from build123d import *

# Parameters (mm, degrees)
SKETCH_W        = 40
SKETCH_H        = 42
SKETCH_R        = 1.6
PAD_DEPTH       = 12
SKETCH001_R     = 4.075
POCKET_DEPTH    = 42.001
SKETCH003_R     = 1.6
PAD001_DEPTH    = 40
SKETCH004_W     = 8.15
SKETCH004_H     = 42
SKETCH004_R     = 3
SKETCH004_W_2   = 7.5
POCKET001_DEPTH = 10.001
POCKET002_DEPTH = 3
POCKET003_DEPTH = 3
FILLET_R        = 4
FILLET001_R     = 3
SKETCH008_R     = 1.6
POCKET004_DEPTH = 40.001
POCKET005_DEPTH = 3
POCKET006_DEPTH = 3
POCKET007_DEPTH = 40.001


with BuildPart() as part:
    # Sketch → Pad (new body)
    with BuildSketch(Plane.XY):
        Rectangle(SKETCH_W, SKETCH_H)
        with Locations((-14.85, 11.875)):
            Circle(SKETCH_R, mode=Mode.SUBTRACT)
        with Locations((14.85, 11.875)):
            Circle(SKETCH_R, mode=Mode.SUBTRACT)
        with Locations((-14.85, -11.875)):
            Circle(SKETCH_R, mode=Mode.SUBTRACT)
        with Locations((14.85, -11.875)):
            Circle(SKETCH_R, mode=Mode.SUBTRACT)
    extrude(amount=PAD_DEPTH)

    # Sketch001 (on Face3 of Pad) → Pocket (cut, through all)
    with BuildSketch(Plane.XZ.offset(21)):
        with Locations((0, 6)):
            Circle(SKETCH001_R)
    extrude(amount=-POCKET_DEPTH, mode=Mode.SUBTRACT)

    # Sketch003 (on Face2 of Pocket) → Pad001 (join)
    with BuildSketch(Plane(origin=(-20, 0, 0), x_dir=(0, -1, 0), z_dir=(-1, 0, 0))):
        with BuildLine():
            ThreePointArc((16.875, 17), (11.875, 22), (6.875, 17))
            Line((6.875, 17), (6.875, 12))
            Line((16.875, 12), (6.875, 12))
            Line((16.875, 12), (16.875, 17))
        make_face()
        with Locations((11.875, 17)):
            Circle(SKETCH003_R, mode=Mode.SUBTRACT)
    extrude(amount=-PAD001_DEPTH)

    # Sketch004 (on Face4 of Pad001) → Pocket001 (cut, through all)
    with BuildSketch(Plane.XY.offset(12)):
        with Locations((-15.925, 0)):
            Rectangle(SKETCH004_W, SKETCH004_H)
        with Locations((-14.85, 11.875)):
            Circle(SKETCH004_R, mode=Mode.SUBTRACT)
        with Locations((15.925, 0)):
            Rectangle(SKETCH004_W, SKETCH004_H)
        Rectangle(SKETCH004_W_2, SKETCH004_H)
    extrude(amount=POCKET001_DEPTH, mode=Mode.SUBTRACT)

    # Sketch005 (on Face31 of Pocket001) → Pocket002 (cut)
    with BuildSketch(Plane.YZ.offset(11.85)):
        Polygon((-10.258419, 19.8), (-13.491581, 19.8), (-15.108162, 17), (-13.491581, 14.2), (-10.258419, 14.2), (-8.641838, 17), align=None)
    extrude(amount=-POCKET002_DEPTH, mode=Mode.SUBTRACT)

    # Sketch006 (on Face27 of Pocket002) → Pocket003 (cut)
    with BuildSketch(Plane(origin=(-11.85, 0, 0), x_dir=(0, -1, 0), z_dir=(-1, 0, 0))):
        Polygon((13.491581, 19.8), (10.258419, 19.8), (8.641838, 17), (10.258419, 14.2), (13.491581, 14.2), (15.108162, 17), align=None)
    extrude(amount=-POCKET003_DEPTH, mode=Mode.SUBTRACT)

    # Fillet
    fillet_edges = [part.edges().sort_by_distance(p)[0] for p in [
        (7.8, -16.875, 12),
        (-7.8, -16.875, 12),
        (7.8, -6.875, 12),
        (-7.8, -6.875, 12),
    ]]
    fillet(fillet_edges, radius=FILLET_R)

    # Fillet001
    fillet001_edges = [part.edges().sort_by_distance(p)[0] for p in [
        (20, -21, 6),
        (-20, -21, 6),
        (20, 21, 6),
        (-20, 21, 6),
    ]]
    fillet(fillet001_edges, radius=FILLET001_R)

    # Sketch008 (on Face5 of Fillet001) → Pocket004 (cut, through all)
    with BuildSketch(Plane(origin=(-20, 0, 0), x_dir=(0, -1, 0), z_dir=(-1, 0, 0))):
        with Locations((-4, 6)):
            Circle(SKETCH008_R)
        with Locations((4, 6)):
            Circle(SKETCH008_R)
    extrude(amount=-POCKET004_DEPTH, mode=Mode.SUBTRACT)

    # Sketch009 (on Face5 of Pocket004) → Pocket005 (cut)
    with BuildSketch(Plane(origin=(-20, 0, 0), x_dir=(0, -1, 0), z_dir=(-1, 0, 0))):
        Polygon((-2.383419, 8.8), (-5.616581, 8.8), (-7.233162, 6), (-5.616581, 3.2), (-2.383419, 3.2), (-0.766838, 6), align=None)
        Polygon((5.616581, 8.8), (2.383419, 8.8), (0.766838, 6), (2.383419, 3.2), (5.616581, 3.2), (7.233162, 6), align=None)
    extrude(amount=-POCKET005_DEPTH, mode=Mode.SUBTRACT)

    # Sketch010 (on Face42 of Pocket005) → Pocket006 (cut)
    with BuildSketch(Plane.YZ.offset(20)):
        Polygon((-2.383419, 8.8), (-5.616581, 8.8), (-7.233162, 6), (-5.616581, 3.2), (-2.383419, 3.2), (-0.766838, 6), align=None)
        Polygon((5.616581, 8.8), (2.383419, 8.8), (0.766838, 6), (2.383419, 3.2), (5.616581, 3.2), (7.233162, 6), align=None)
    extrude(amount=-POCKET006_DEPTH, mode=Mode.SUBTRACT)

    # Sketch008 (on Face5 of Fillet001) → Pocket007 (cut, through all)
    with BuildSketch(Plane(origin=(-20, 0, 0), x_dir=(0, -1, 0), z_dir=(-1, 0, 0))):
        with Locations((-4, 6)):
            Circle(SKETCH008_R)
        with Locations((4, 6)):
            Circle(SKETCH008_R)
    extrude(amount=-POCKET007_DEPTH, mode=Mode.SUBTRACT)


solid = part.part
The listing builds one solid part. Answer for the finished solid, in the listing's coordinates (mm). A direction names the side the tool comes from. Give positions to 0.01 mm unless a question says otherwise; leave off trailing zeros. Loops run counter-clockwise (first coordinate to the right, second up) from the corner with the lowest first, then second, coordinate; pieces in that order, holes last. Notation, with made-up numbers: (9.5, 48) - (27.5, 48) arc R11 ccw to (27.5, 63) - close; hole circle Ø11 at (-34, 10). An arc over 180 degrees is marked (long way). Write each question's results on one line, items separated by ' | '.
1. For a pull along Y with two mould halves and no side action, classify faces 1 (the face through (-20, 0, 6)), 2 (the face through (-4, 21, 4.6)), 3 (the face through (16.376, 12.356, 5.916)) as +Y half, -Y half, draft (parallel to the pull), parting line (faces both ways), or undercut.
Resolved:
face 1: draft | face 2: +Y half | face 3: undercut
2. Which of the six approach directions +Z, -Z, +X, -X, +Y, -Y give full straight-line access (tool end or side, diameter ignored) to faces 4 (the face through (10.4, -14.3, 15.6)), 5 (the face through (-18.521, 6.436, 4.62)), 6 (the face through (-3.75, -12, 15)), 7 (the face through (11.85, -14, 14.7))?
Resolved:
face 4: +X | face 5: -X | face 6: +Z, +Y, -Y | face 7: +Z, +X, +Y, -Y
3. Find section C-C, the plane x = 0. Write down the section's boundary in (y, z) (3 decimals).
Resolved:
outline: (-21, 0) - (21, 0) - (21, 1.925) - (-21, 1.925) - close; (-21, 10.075) - (21, 10.075) - (21, 12) - (-21, 12) - close
4. Find section A-A, the plane x = 14.85. Write down the section's boundary in (y, z) (3 decimals).
Resolved:
outline: (-21, 0) - (-13.475, 0) - (-13.475, 12) - (-21, 12) - close; (-10.275, 0) - (10.275, 0) - (10.275, 12) - (-10.275, 12) - close; (13.475, 0) - (21, 0) - (21, 12) - (13.475, 12) - close; hole circle Ø3.2 at (-4, 6); hole circle Ø3.2 at (4, 6)
5. Consider probe 1 along Y at (x, z) = (14.85, 8) (3 decimals); probe 2 along Y at (x, z) = (9, 6); probe 3 along Y at (x, z) = (14.85, 6) (3 decimals). Determine where each line is inside the solid, lowest interval first. Write a range as from..to.
Resolved:
probe 1: y = -21..-13.475, -10.275..10.275, 13.475..21 | probe 2: y = -21..-5.6, -2.4..2.4, 5.6..21 | probe 3: y = -21..-13.475, -10.275..-5.6, -2.4..2.4, 5.6..10.275, 13.475..21
6. Flat-ended cylindrical pins translate along their axes: P1, Ø11, axis at y = -10.5, z = 16, coming from the +X side; P2, Ø4, axis at y = -11.875, z = 17, coming from the +X side; P3, Ø0.5, axis at x = 6, z = 16.5, coming from the -Y side (3 decimals); P4, Ø0.9, axis at x = 18.5, y = 4, coming from the +Z side. Find the tip coordinate at first contact, or state that the pin passes through.
Resolved:
P1: stops at x = 20 | P2: stops at x = 8.85 | P3: stops at y = -16.875 | P4: stops at z = 12
7. Find section B-B, the plane y = 4. Write down the section's boundary in (x, z) (3 decimals), then the cut area to 3 significant figures.
Resolved:
outline: (-20, 0) - (20, 0) - (20, 3.2) - (17, 3.2) - (17, 4.4) - (3.748, 4.4) arc R4.075 cw to (-3.748, 4.4) - (-17, 4.4) - (-17, 3.2) - (-20, 3.2) - close; (-20, 8.8) - (-17, 8.8) - (-17, 7.6) - (-3.748, 7.6) arc R4.075 cw to (3.748, 7.6) - (17, 7.6) - (17, 8.8) - (20, 8.8) - (20, 12) - (-20, 12) - close | area: 311 mm^2
8. Find section D-D, the plane y = 11. Write down the section's boundary in (x, z) (3 decimals).
Resolved:
outline: (-20, 0) - (-16.19, 0) - (-16.19, 12) - (-20, 12) - close; (-13.51, 0) - (13.51, 0) - (13.51, 12) - (-13.51, 12) - close; (16.19, 0) - (20, 0) - (20, 12) - (16.19, 12) - close; hole circle Ø8.15 at (0, 6)
